Verification items for the finished model (mm, model axes). Face numbers are marked on the shaded views. A direction names the side the tool comes from. Give positions to 0.01 mm unless a question says otherwise; leave off trailing zeros. Order: outer loops, then holes, each group sorted by start corner. A loop starts at its lowest first (then second) coordinate and runs counter-clockwise, first axis right, second up. Notation, with made-up numbers: (47, 46.25) - (100, 46.25) arc R22 ccw to (100, 66.25) - close; hole circle Ø11 at (40, 68). An arc over 180 degrees is marked (long way). Answer as a JSON object with one key per item and string values.
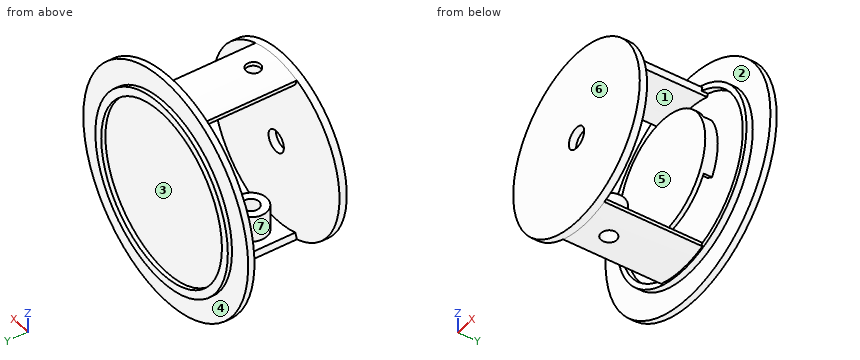
```python
from build123d import *

# Parameters (mm, degrees)
F0_R           = 28
F1_DEPTH       = 1.5
F3_DEPTH       = 5.1
F5_DEPTH       = 25
F6_R           = 21.5
F7_DEPTH       = 1.75
F8_R           = 2.6
F9_DEPTH       = 25
F10_R          = 1.975
F11_DEPTH      = 30
F13_END_RADIUS = 21.5
F12_R          = 3.75
F12_R_2        = 1.875
F13_REACH      = 38.6076017178
F14_W          = 15
F14_H          = 26.820743024
F15_DEPTH      = 25
F15_DEPTH_BACK = 25
F16_R          = 14.5
F17_DEPTH      = 1
F19_DEPTH      = 2
F21_R          = 22.5
F21_R_2        = 20.5
F22_DEPTH      = 1
F23_R          = 22
F23_R_2        = 20.75
F24_DEPTH      = 1.5
F25_R          = 3.1
F26_DEPTH      = 5.5
F27_R          = 1.75
F28_REACH      = 12.4507474683
F29_R          = 30
F29_R_2        = 29
F30_DEPTH      = 25


with BuildPart() as f1:
    # F0 (on Front) → F1 (new body)
    with BuildSketch(Plane.XZ):
        Circle(F0_R)
    extrude(amount=F1_DEPTH)

    # F2 (on face) → F3 (join)
    with BuildSketch(Plane.XZ.offset(1.5)):
        with BuildLine():
            ThreePointArc((0, -13), (-13, 0), (0, 13))
            Line((0, 13), (0, 14.5))
            ThreePointArc((0, 14.5), (-14.5, 0), (0, -14.5))
            Line((0, -14.5), (0, -13))
        make_face()
    extrude(amount=F3_DEPTH)

    # F4 (on face) → F5 (join)
    with BuildSketch(Plane.XZ.offset(1.5)):
        with BuildLine():
            Line((6.5113630891, 18.910371512), (6.9997153208, 20.3286493754))
            ThreePointArc((6.9997153208, 20.3286493754), (0, 21.5), (-6.9997153208, 20.3286493754))
            Line((-6.9997153208, 20.3286493754), (-6.5113630891, 18.910371512))
            ThreePointArc((-6.5113630891, 18.910371512), (0, 20), (6.5113630891, 18.910371512))
        make_face()
        with BuildLine():
            ThreePointArc((6.5113630891, -18.910371512), (0, -20), (-6.5113630891, -18.910371512))
            Line((-6.5113630891, -18.910371512), (-6.9997153208, -20.3286493754))
            ThreePointArc((-6.9997153208, -20.3286493754), (0, -21.5), (6.9997153208, -20.3286493754))
            Line((6.9997153208, -20.3286493754), (6.5113630891, -18.910371512))
        make_face()
    extrude(amount=F5_DEPTH)

    # F6 (on face) → F7 (join)
    with BuildSketch(Plane.XZ.offset(26.5)):
        Circle(F6_R)
    extrude(amount=F7_DEPTH)

    # F8 (on face) → F9 (cut)
    with BuildSketch(Plane.XZ.offset(28.25)):
        Circle(F8_R)
    extrude(amount=-F9_DEPTH, mode=Mode.SUBTRACT)

    # F10 (on Top) → F11 (cut)
    with BuildSketch(Plane.XY):
        with Locations((0, -20.5)):
            Circle(F10_R)
    extrude(amount=-F11_DEPTH, mode=Mode.SUBTRACT)

    f13_end = (Plane.ZX.offset(-14) * Cylinder(F13_END_RADIUS, 245.3825308212, mode=Mode.PRIVATE)).faces().sort_by_distance((0, -14, -21.5))[0]
    # F12 (on Top) → F13 (join, up to the whole of a round face its end follows)
    with BuildSketch(Plane.XY):
        with Locations((0, -20.5)):
            Circle(F12_R)
        with Locations((0, -20.5)):
            Circle(F12_R_2, mode=Mode.SUBTRACT)
    f13_long = extrude(amount=-F13_REACH, mode=Mode.PRIVATE)
    add(split(f13_long, bisect_by=f13_end, keep=Keep.BOTTOM, mode=Mode.PRIVATE))

    # F14 (on Right) → F15 (cut, two sides)
    with BuildSketch(Plane.YZ) as f15_sk:
        with Locations((-17.75, 0)):
            Rectangle(F14_W, F14_H)
    extrude(amount=-F15_DEPTH, mode=Mode.SUBTRACT)
    extrude(f15_sk.sketch, amount=F15_DEPTH_BACK, mode=Mode.SUBTRACT)

    # F16 (on face) → F17 (join)
    with BuildSketch(Plane.XZ.offset(6.6)):
        Circle(F16_R)
    extrude(amount=F17_DEPTH)

    # F18 (on face) → F19 (join)
    with BuildSketch(Plane(origin=(0, -6.6, 0), x_dir=(-1, 0, 0), z_dir=(0, 1, 0))):
        with BuildLine():
            Line((-11.0418238983, 6.375), (-12.5573683549, 7.25))
            ThreePointArc((-12.5573683549, 7.25), (-14.5, 0), (-12.5573683549, -7.25))
            Line((-12.5573683549, -7.25), (-11.0418238983, -6.375))
            ThreePointArc((-11.0418238983, -6.375), (-12.75, 0), (-11.0418238983, 6.375))
        make_face()
    extrude(amount=F19_DEPTH)

    # F21 (on face) → F22 (join)
    with BuildSketch(Plane(origin=(0, 0, 0), x_dir=(-1, 0, 0), z_dir=(0, 1, 0))):
        Circle(F21_R)
        Circle(F21_R_2, mode=Mode.SUBTRACT)
    extrude(amount=F22_DEPTH)

    # F23 (on face) → F24 (join)
    with BuildSketch(Plane.XZ.offset(1.5)):
        Circle(F23_R)
        Circle(F23_R_2, mode=Mode.SUBTRACT)
    extrude(amount=F24_DEPTH)

    # F25 (on offset) → F26 (cut)
    with BuildSketch(Plane.XY.offset(15)):
        with Locations((0, -21)):
            Circle(F25_R)
    extrude(amount=F26_DEPTH, mode=Mode.SUBTRACT)

    f28_end = f1.faces().sort_by_distance((17.5034836447, -27.1584498842, 12.4851135478))[0]
    # F27 (on face) → F28 (cut, up to a face of the model that its end follows)
    with BuildSketch(Plane(origin=(0, 0, 20.5), x_dir=(1, 0, 0), z_dir=(0, 0, -1))):
        with Locations((0, 21)):
            Circle(F27_R)
    f28_long = extrude(amount=-F28_REACH, mode=Mode.PRIVATE)
    add(split(f28_long, bisect_by=f28_end, keep=Keep.BOTTOM, mode=Mode.PRIVATE), mode=Mode.SUBTRACT)

    # F29 (on face) → F30 (cut)
    with BuildSketch(Plane.XZ.offset(1.5)):
        Circle(F29_R)
        Circle(F29_R_2, mode=Mode.SUBTRACT)
    extrude(amount=F30_DEPTH, mode=Mode.SUBTRACT)


solid = f1.part
```
(1) Gauge pin test, flat ends, axial feed: pin 1 Ø3 at (x, z) = (12, 2.5) entering from +Y; pin 2 Ø12 at (x, y) = (-4.5, -23) entering from +Z; pin 3 Ø1.9 at (x, y) = (-1, -21.5) entering from -Z. Record the tip position at first contact, or that the pin passes through.
Computed values:
{"pin 1": "stops at y = 0", "pin 2": "stops at z = 21.5", "pin 3": "stops at z = -21.49"}
(2) Release check for a two-part mould opening along Y. For the marked faces 1, 2 and 3 record: pulls with the +Y half, pulls with the -Y half, needs draft (parallel to the pull), parting line crosses it, or undercut.
Computed values:
{"face 1": "undercut", "face 2": "pulls with the -Y half", "face 3": "pulls with the +Y half"}
(3) Section check A-A (y = -11.25). Record the cut outline in (x, z).
Computed values:
{"outline": "(-7, -20.33) arc R21.5 ccw to (7, -20.33) - (6.51, -18.91) arc R20 cw to (-6.51, -18.91) - close; (-7, 20.33) - (-6.51, 18.91) arc R20 cw to (6.51, 18.91) - (7, 20.33) arc R21.5 ccw to start"}
(4) Access from +Z, -Z, +X, -X, +Y, -Y to the whole of each face (thin tool, end or side, straight path). Record for the marked faces 4, 5, 6 and 7.
Computed values:
{"face 4": "+Y", "face 5": "+X, -X", "face 6": "+Z, -Z, +X, -X, -Y", "face 7": "none"}
(5) Section check D-D (z = 0). Count the separate pieces of the cut face and the enclosed holes in it, then the cut area to 3 significant figures.
Computed values:
{"separate pieces": "3", "enclosed holes": "0", "area": "198 mm²"}
(6) Section check C-C (x = -18). Record the cut outline in (y, z), then the cut area to 3 significant figures.
Computed values:
{"outline": "(-28.25, -11.76) - (-26.5, -11.76) - (-26.5, 11.76) - (-28.25, 11.76) - close; (-3, -12.65) - (-1.5, -12.65) - (-1.5, -21.45) - (0, -21.45) - (0, -13.5) - (1, -13.5) - (1, -9.81) - (0, -9.81) - (0, 9.81) - (1, 9.81) - (1, 13.5) - (0, 13.5) - (0, 21.45) - (-1.5, 21.45) - (-1.5, 12.65) - (-3, 12.65) - (-3, 10.32) - (-1.5, 10.32) - (-1.5, -10.32) - (-3, -10.32) - close", "area": "120 mm²"}
(7) Material ranges on line 1 along Y through (x, z) = (0, -18.25) (3 decimals); line 2 along Z through (x, y) = (0, 0.65); line 3 along Y through (x, z) = (-8, -7.5), recorded low to high. Write a range as [from, to].
Computed values:
{"line 1": "y = [-28.25, -26.5], [-24.25, -22.375], [-18.625, -16.75], [-1.5, 0]", "line 2": "z = [-22.5, -20.5], [20.5, 22.5]", "line 3": "y = [-28.25, -26.5], [-7.6, -6.6], [-1.5, 0]"}
